```python
from build123d import *

# Parameters (mm, degrees)
F0_W     = 127
F0_H     = 101.6
F1_DEPTH = 15.875
F3_DEPTH = 19.05
F5_DEPTH = 15.875
F6_R     = 50.8


with BuildPart() as f1:
    # F0 (on Front) → F1 (new body)
    with BuildSketch(Plane.XZ):
        with Locations((-62.0965630407, -41.252563009)):
            Rectangle(F0_W, F0_H)
    extrude(amount=F1_DEPTH)

    # F2 (on face) → F3 (cut)
    with BuildSketch(Plane.XZ.offset(15.875)):
        with BuildLine():
            Line((-1.0253972141, -92.052563009), (1.4034369593, -92.052563009))
            Line((1.4034369593, -92.052563009), (1.4034369593, -80.1284596617))
            ThreePointArc((1.4034369593, -80.1284596617), (0.6228444874, -86.1788775646), (-1.0253972141, -92.052563009))
        make_face()
        with BuildLine():
            Line((1.4034369593, -75.45119524), (1.4034369593, -80.1284596617))
            ThreePointArc((1.4034369593, -80.1284596617), (1.4685491276, -77.7898274509), (1.4034369593, -75.45119524))
        make_face()
    extrude(amount=-F3_DEPTH, mode=Mode.SUBTRACT)

    # F4 (on face) → F5 (join)
    with BuildSketch(Plane.XZ.offset(15.875)):
        with BuildLine():
            Line((-1.0253972141, -92.052563009), (-125.5965630407, -92.052563009))
            Line((-125.5965630407, -92.052563009), (-139.2145454884, -128.8291364908))
            Line((-139.2145454884, -128.8291364908), (-44.9651107192, -170.3518033028))
            Line((-44.9651107192, -170.3518033028), (-5.2652601153, -102.3738086224))
            ThreePointArc((-5.2652601153, -102.3738086224), (-2.7865893027, -97.3605523032), (-1.0253972141, -92.052563009))
        make_face()
    extrude(amount=-F5_DEPTH)

    # F6
    f6_edges = [f1.edges().sort_by_distance(p)[0] for p in [
        (-125.596563, -7.9375, -92.052563),
    ]]
    fillet(f6_edges, radius=F6_R)


solid = f1.part
```
Verification items for the finished model (mm, model axes). A direction names the side the tool comes from. Coordinates: 2 decimals unless noted, no trailing zeros. Order: outer loops, then holes, each group sorted by start corner. A loop starts at its lowest first (then second) coordinate and runs counter-clockwise, first axis right, second up. Notation, with made-up numbers: (62.25, 7) -> (88.25, 7) arc R22 ccw to (88.25, 19) -> close; hole circle Ø9 at (33.5, -5). An arc over 180 degrees is marked (long way). Answer as CSV lines item,"result". Start each with the question number.
1) Gauge pin test, flat ends, axial feed: pin 1 Ø5 at (y, z) = (-7.5, -128) entering from -X; pin 2 Ø3 at (y, z) = (-13.5, -103.5) entering from +X; pin 3 Ø5 at (y, z) = (-10, -139.5) entering from -X; pin 4 Ø8 at (x, y) = (-125, -11) entering from -Z. Record the tip position at first contact, or that the pin passes through.
2) Cross-section at B-B, the plane z = -126.5. Record the boundary of the cut face in (x, y) (3 decimals).
3) Cross-section at C-C, the plane x = -82.5. Record the boundary of the cut face in (y, z) (3 decimals).
4) Set-up check for faces 1 (the face through (0.64, -8.05, -86.1)), 2 (the face through (-125.597, -8, -37)): record each of +Z, -Z, +X, -X, +Y, -Y from which the full face is reachable in a straight line by a thin tool's end or side.
5) Material ranges on L1, parallel to X at y = -6, z = -35; L2, parallel to X at y = -9, z = -113.5; L3, parallel to Z at x = -103, y = -2.25, recorded low to high. Write a range as [from, to].
6) Cross-section at A-A, the plane y = -6.75. Record the boundary of the cut face in (x, z).
Conclusion:
1,pin 1,"stops at x = -139.21"
1,pin 2,"stops at x = -5.05"
1,pin 3,"stops at x = -120.67"
1,pin 4,"stops at z = -136.85"
2,outline,"(-138.352, -15.875) -> (-19.355, -15.875) -> (-19.355, 0) -> (-138.352, 0) -> close"
3,outline,"(-15.875, -153.815) -> (0, -153.815) -> (0, 9.547) -> (-15.875, 9.547) -> close"
4,face 1,"-Z, +X, +Y, -Y"
4,face 2,"+Z, -X, +Y, -Y"
5,L1,"x = [-125.6, 1.4]"
5,L2,"x = [-133.54, -11.76]"
5,L3,"z = [-144.78, 9.55]"
6,outline,"(-139.21, -128.83) -> (-44.97, -170.35) -> (-5.27, -102.37) arc R40.32 ccw to (-1.03, -92.05) arc R42.03 ccw to (1.4, -80.13) -> (1.4, 9.55) -> (-125.6, 9.55) -> (-125.6, -82.95) arc R50.8 cw to (-128.76, -100.59) -> close"
